from build123d import *

# Parameters (mm, degrees)
BOSS_EXTRUDE1_DEPTH = 56.896
FILLET1_R           = 2.54
FILLET2_R           = 2.54
SKETCH2_R           = 9.652
BOSS_EXTRUDE2_DEPTH = 8.2804
SKETCH3_R           = 5.08
BOSS_EXTRUDE3_DEPTH = 13.716


with BuildPart() as part:
    # Sketch1 → Boss-Extrude1 (new body)
    with BuildSketch(Plane(origin=(0, 0, 0), x_dir=(0, 0, -1), z_dir=(1, 0, 0))):
        with BuildLine():
            Line((-11.019402446, 14.732), (11.019402446, 14.732))
            ThreePointArc((11.019402446, 14.732), (17.9705, 0), (11.019402446, -14.732))
            Line((11.019402446, -14.732), (-11.019402446, -14.732))
            ThreePointArc((-11.019402446, -14.732), (-17.9705, 0), (-11.019402446, 14.732))
        make_face()
    extrude(amount=BOSS_EXTRUDE1_DEPTH)

    # Fillet1
    fillet1_edges = [part.edges().sort_by_distance(p)[0] for p in [
        (28.448, -14.732, -11.019402446),
        (28.448, -14.732, 11.019402446),
    ]]
    fillet(fillet1_edges, radius=FILLET1_R)

    # Fillet2
    fillet2_edges = [part.edges().sort_by_distance(p)[0] for p in [
        (28.448, 14.732, 11.019402446),
        (28.448, 14.732, -11.019402446),
    ]]
    fillet(fillet2_edges, radius=FILLET2_R)

    # Sketch2 → Boss-Extrude2 (add)
    with BuildSketch(Plane.ZY):
        with Locations(Location((0, 0, 0), (0, 0, 180))):
            Circle(SKETCH2_R)
    extrude(amount=BOSS_EXTRUDE2_DEPTH)

    # Sketch3 → Boss-Extrude3 (add)
    with BuildSketch(Plane.ZY.offset(8.2804)):
        Circle(SKETCH3_R)
    extrude(amount=BOSS_EXTRUDE3_DEPTH)


solid = part.part
The listing builds one solid part. Answer for the finished solid, in the listing's coordinates (mm). A direction names the side the tool comes from. Give positions to 0.01 mm unless a question says otherwise; leave off trailing zeros. Order: outer loops, then holes, each group sorted by start corner. A loop starts at its lowest first (then second) coordinate and runs counter-clockwise, first axis right, second up. Notation, with made-up numbers: (18.25, 67.5) -> (50.25, 67.5) arc R25 cw to (50.25, 81.5) -> close; hole circle Ø8 at (-9.75, 7). An arc over 180 degrees is marked (long way). Put each result on its own line as item: value.
Item 1: A cutting plane is placed at A-A on z = 0. Give the vertices of the cut face in (x, y).
Established:
outline: (-22, -5.08) -> (-8.28, -5.08) -> (-8.28, -9.65) -> (0, -9.65) -> (0, -14.73) -> (56.9, -14.73) -> (56.9, 14.73) -> (0, 14.73) -> (0, 9.65) -> (-8.28, 9.65) -> (-8.28, 5.08) -> (-22, 5.08) -> close
Item 2: For faces 1 (the face through (0, 10, 0)), 2 (the face through (28.846, 14.554, -11.005)), determine the directions among +Z, -Z, +X, -X, +Y, -Y from which every point of the face is accessible in a straight line to the end or side of a thin tool.
Established:
face 1: -X
face 2: -Z, +X, -X, +Y
Item 3: Straight lines are drawn through the part: line 1 (X direction, y = 6.25, z = -12); line 2 (X direction, y = -3.75, z = -4.5); line 3 (Z direction, x = 17.5, y = -7). For each, find the intervals that lie inside material, in ascending order.
Established:
line 1: x = 0 to 56.9
line 2: x = -8.28 to 56.9
line 3: z = -16.64 to 16.64
Item 4: A cutting plane is placed at B-B on y = 0. Give the vertices of the cut face in (x, z).
Established:
outline: (-22, -5.08) -> (-8.28, -5.08) -> (-8.28, -9.65) -> (0, -9.65) -> (0, -17.97) -> (56.9, -17.97) -> (56.9, 17.97) -> (0, 17.97) -> (0, 9.65) -> (-8.28, 9.65) -> (-8.28, 5.08) -> (-22, 5.08) -> close
Item 5: Given P1, Ø1, axis at x = 18.5, y = -7, coming from the +Z side; P2, Ø12, axis at x = 43, z = -12.5, coming from the +Y side; P3, Ø1.5, axis at x = 47.5, y = 4, coming from the +Z side; P4, Ø2, axis at x = -7, y = 5, coming from the +Z side, each flat-ended and moving along its own axis, determine where each tip first touches the part or whether it passes through.
Established:
P1: stops at z = 16.83
P2: stops at y = 14.73
P3: stops at z = 17.69
P4: stops at z = 8.78
Item 6: A cutting plane is placed at C-C on x = 20. Give the vertices of the cut face in (y, z).
Established:
outline: (-14.73, -10.07) arc R2.54 ccw to (-14.06, -11.79) arc R19.09 ccw to (14.06, -11.79) arc R2.54 ccw to (14.73, -10.07) -> (14.73, 10.07) arc R2.54 ccw to (14.06, 11.79) arc R19.09 ccw to (-14.06, 11.79) arc R2.54 ccw to (-14.73, 10.07) -> close
Item 7: A cutting plane is placed at D-D on z = -8. Give the vertices of the cut face in (x, y), plus the area to 3 significant figures.
Established:
outline: (-8.28, -5.4) -> (0, -5.4) -> (0, -14.73) -> (56.9, -14.73) -> (56.9, 14.73) -> (0, 14.73) -> (0, 5.4) -> (-8.28, 5.4) -> close
area: 1,770 mm^2
